Autodesk Inventor part; units mm, degrees
ref_plane "YZ Plane" through (0, 0, 0) normal (1, 0, 0) x (0, 1, 0)
ref_plane "XZ Plane" through (0, 0, 0) normal (0, 1, 0) x (-1, 0, 0)
ref_plane "XY Plane" through (0, 0, 0) normal (0, 0, 1) x (1, 0, 0)
sketch "Sketch1" plane through (0, 0, 0) normal (0, 1, 0) x (-1, 0, 0)
  line L0 (0, 0) -> (82.042, 0)
  line L1 (82.042, 0) -> (82.042, -149.606)
  line L2 (82.042, -149.606) -> (0, -149.606)
  line L3 (0, -149.606) -> (0, 0)
  dimension "d0" = 82.042
  dimension "d1" = 149.606
extrude "Extrusion1" add sketch "Sketch1" along normal blind 19.558
fillet "Fillet1" radius 6.35 4 edges at (0, 9.779, 0) (-82.042, 9.779, 0) (-82.042, 9.779, -149.606) (0, 9.779, -149.606)
fillet "Fillet2" radius 3.175 16 edges at (-80.1821, 19.558, -147.7461) (-82.042, 19.558, -74.803) (-80.1821, 19.558, -1.8599) (-41.021, 19.558, 0) (-1.8599, 19.558, -1.8599) (0, 19.558, -74.803) (-1.8599, 19.558, -147.7461) (-41.021, 19.558, -149.606) (-1.8599, 0, -1.8599) (-41.021, 0, 0) (-80.1821, 0, -1.8599) (-82.042, 0, -74.803) (-80.1821, 0, -147.7461) (-41.021, 0, -149.606) (-1.8599, 0, -147.7461) (0, 0, -74.803)
sketch "Sketch2" plane through (-75.692, 3.175, 0) normal (0, 0, 1) x (1, 0, 0)
  line L0 (69.342, 0) -> (0, 0)
  line L1 (69.342, 13.208) -> (69.342, 0)
  line L2 (0, 13.208) -> (69.342, 13.208)
  line L3 (0, 0) -> (0, 13.208)
  line L4 (0, 13.208) -> (0, 0)
  line L5 (0, 6.604) -> (12.7, 6.604)
  line L6 (69.342, 0) -> (69.342, 13.208)
  line L7 (69.342, 6.604) -> (56.642, 6.604)
  line L8 (6.35, 4.064) -> (19.05, 4.064)
  line L9 (19.05, 4.064) -> (19.05, 9.144)
  line L10 (19.05, 9.144) -> (6.35, 9.144)
  line L11 (6.35, 9.144) -> (6.35, 4.064)
  line L12 (6.35, 4.064) -> (19.05, 9.144) construction
  line L13 (19.05, 4.064) -> (6.35, 9.144) construction
  line L14 (50.292, 4.064) -> (62.992, 4.064)
  line L15 (62.992, 4.064) -> (62.992, 9.144)
  line L16 (62.992, 9.144) -> (50.292, 9.144)
  line L17 (50.292, 9.144) -> (50.292, 4.064)
  line L18 (50.292, 4.064) -> (62.992, 9.144) construction
  line L19 (62.992, 4.064) -> (50.292, 9.144) construction
  point P0 (75.692, -3.175)
  dimension "d6" = 12.7
  dimension "d7" = 12.7
  dimension "d8" = 12.7
  dimension "d9" = 5.08
  dimension "d10" = 12.7
  dimension "d11" = 5.08
extrude "Extrusion2" cut sketch "Sketch2" against normal blind 3.175 contours L15 L14 L17 L16 | L11 L10 L9 L8
chamfer "Chamfer1" distance 0.7937 angle 45 8 edges at (-69.342, 9.779, 0) (-62.992, 12.319, 0) (-62.992, 7.239, 0) (-56.642, 9.779, 0) (-25.4, 9.779, 0) (-19.05, 12.319, 0) (-19.05, 7.239, 0) (-12.7, 9.779, 0)
properties part number "Battery"
Geometry: final body of the model. Coordinates: model frame, mm. Coordinates: 2 decimals unless noted, no trailing zeros. Use CSV: the item, a comma, the result in double quotes. Start each with the question number.
1. Ray query, probe 1 along Z at (x, y) = (-23, 9) (3 decimals); probe 2 along X at (y, z) = (16.5, -88.5); probe 3 along X at (y, z) = (1.5, -121). Return the intervals inside material, ascending.
2. Mould query, pull axis Y, two halves, no side actions, for faces 1 (the face through (-40, 0, -74)), 2 (the face through (-81.14, 18.6, -75.76)), 3 (the face through (-63, 10, -3.175)). Classes: pulls with the +Y half, pulls with the -Y half, needs draft (parallel to the pull), parting line crosses it, or undercut.
3. First-contact query: P1, Ø1.5, axis at x = -66, y = 11, coming from the +Z side (3 decimals); P2, Ø1.9, axis at y = 10.5, z = -2.5, coming from the +X side; P3, Ø2.5, axis at x = -64, z = -1.5, coming from the +Y side. Flat tips, straight axial feed; report the tip coordinate or a pass-through.
Entries:
1,probe 1,"-149.606 to -3.175"
1,probe 2,"-82.04 to 0"
1,probe 3,"-81.56 to -0.48"
2,face 1,"pulls with the -Y half"
2,face 2,"pulls with the +Y half"
2,face 3,"undercut"
3,P1,"z = -3.175"
3,P2,"x = -0.7"
3,P3,"y = 19.53"
